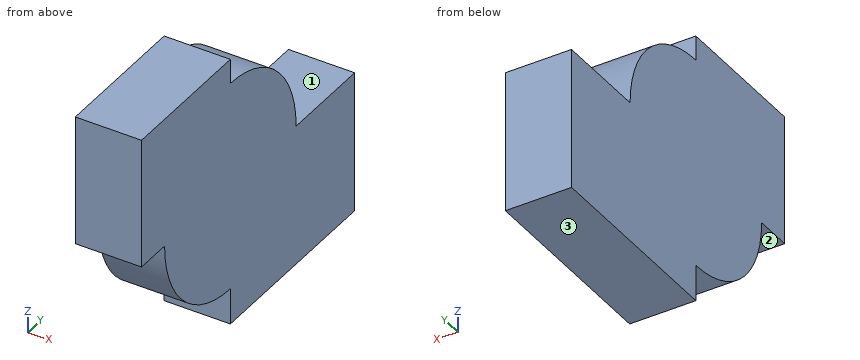
```python
from build123d import *

# Parameters (mm, degrees)
F1_DEPTH = 25.4


with BuildPart() as f1:
    # F0 (on Right) → F1 (new body)
    with BuildSketch(Plane.YZ):
        with BuildLine():
            Line((0, 0), (40.5764031263, 0))
            ThreePointArc((40.5764031263, 0), (28.6918498068, 28.6918498068), (0, 40.5764031263))
            Line((0, 40.5764031263), (0, 0))
        make_face()
        with BuildLine():
            Line((76.691634953, 0), (40.5764031263, 0))
            ThreePointArc((40.5764031263, 0), (28.6918498068, -28.6918498068), (0, -40.5764031263))
            Line((0, -40.5764031263), (0, -54.5102506876))
            Line((0, -54.5102506876), (76.691634953, -54.5102506876))
            Line((76.691634953, -54.5102506876), (76.691634953, 0))
        make_face()
        with BuildLine():
            ThreePointArc((0, -40.5764031263), (28.6918498068, -28.6918498068), (40.5764031263, 0))
            Line((40.5764031263, 0), (0, 0))
            Line((0, 0), (0, -40.5764031263))
        make_face()
        with BuildLine():
            Line((0, 0), (0, 40.5764031263))
            ThreePointArc((0, 40.5764031263), (-28.6918498068, 28.6918498068), (-40.5764031263, 0))
            Line((-40.5764031263, 0), (0, 0))
        make_face()
        with BuildLine():
            ThreePointArc((-40.5764031263, 0), (-28.6918498068, 28.6918498068), (0, 40.5764031263))
            Line((0, 40.5764031263), (0, 50.0971861184))
            Line((0, 50.0971861184), (-54.7840930521, 50.0971861184))
            Line((-54.7840930521, 50.0971861184), (-54.7840930521, 0))
            Line((-54.7840930521, 0), (-40.5764031263, 0))
        make_face()
        with BuildLine():
            ThreePointArc((-40.5764031263, 0), (-28.6918498068, -28.6918498068), (0, -40.5764031263))
            Line((0, -40.5764031263), (0, 0))
            Line((0, 0), (-40.5764031263, 0))
        make_face()
    extrude(amount=F1_DEPTH)


solid = f1.part
```
Can you work these out from the model? Positions are in its coordinate system, mm. Face numbers are marked on the shaded views. A direction names the side the tool comes from. Round coordinates to 2 decimals unless told otherwise and drop trailing zeros. Loops run counter-clockwise (first coordinate to the right, second up) from the corner with the lowest first, then second, coordinate; pieces in that order, holes last. Notation, with made-up numbers: (6.5, 16) -> (14.5, 16) arc R5 cw to (14.5, 24) -> close; hole circle Ø4 at (23, 61.5). An arc over 180 degrees is marked (long way). One line per item, written item: value. Start each with the question number.
1. If we section it at A-A, the plane x = 1.75: Write out the boundary of the cut face in (y, z).
2. For the marked faces 1, 2 and 3, which set-ups out of +Z, -Z, +X, -X, +Y, -Y let a thin tool reach every point of the face, with its end or its side?
3. If I drill on probe 1 along Y at (x, z) = (19, -50); probe 2 along Z at (x, y) = (19.25, 41); probe 3 along Y at (x, z) = (3.5, 44), over which ranges is the centre line in solid material (lowest first)?
4. If we section it at C-C, the plane y = 64.5: Write out the boundary of the cut face in (x, z), then the cut area to 3 significant figures.
5. For pin 1 (3 mm diameter, centred on x = 19, z = 46, fed in from +Y); pin 2 (7 mm diameter, centred on x = 10, y = -46, fed in from -Z); pin 3 (4 mm diameter, centred on x = 9, y = 29.5, fed in from +Z), each with a flat end and sliding along its axis, tell me the tip position at first contact or that it passes through.
6. If we section it at B-B, the plane z = -44.5: Write out the boundary of the cut face in (x, y), then the cut area to 3 significant figures.
Calculated:
1. outline: (-54.78, 0) -> (-40.58, 0) arc R40.58 ccw to (0, -40.58) -> (0, -54.51) -> (76.69, -54.51) -> (76.69, 0) -> (40.58, 0) arc R40.58 ccw to (0, 40.58) -> (0, 50.1) -> (-54.78, 50.1) -> close
2. face 1: +Z, +X, -X, +Y
2. face 2: -Z, +X, -X, -Y
2. face 3: -Z, +X, -X, +Y, -Y
3. probe 1: y = 0 to 76.69
3. probe 2: z = -54.51 to 0
3. probe 3: y = -54.78 to 0
4. outline: (0, -54.51) -> (25.4, -54.51) -> (25.4, 0) -> (0, 0) -> close
4. area: 1,380 mm²
5. pin 1: stops at y = 0
5. pin 2: stops at z = 0
5. pin 3: stops at z = 29.84
6. outline: (0, 0) -> (25.4, 0) -> (25.4, 76.69) -> (0, 76.69) -> close
6. area: 1,950 mm²
